Autodesk Inventor part; units mm, degrees
ref_plane "YZ Plane" through (0, 0, 0) normal (1, 0, 0) x (0, 1, 0)
ref_plane "XZ Plane" through (0, 0, 0) normal (0, 1, 0) x (-1, 0, 0)
ref_plane "XY Plane" through (0, 0, 0) normal (0, 0, 1) x (1, 0, 0)
sketch "Sketch2" plane through (0, 0, 0) normal (0, 0, 1) x (1, 0, 0)
  line L0 (-12.7, -30.6388) -> (12.7, -30.6388)
  line L1 (12.7, -30.6388) -> (12.7, 30.6388)
  line L2 (12.7, 30.6388) -> (-12.7, 30.6388)
  line L3 (-12.7, 30.6388) -> (-12.7, -30.6388)
  line L4 (-12.7, -30.6388) -> (12.7, 30.6388) construction
  line L5 (12.7, -30.6388) -> (-12.7, 30.6388) construction
  line L6 (0, 30.6388) -> (0, -30.6388) construction
  point P0 (0, 0)
  dimension "d0" = 25.4
  dimension "d1" = 61.2775
extrude "Extrusion1" add sketch "Sketch2" along normal blind 25.4
sketch "Sketch3" plane through (0, 0, 25.4) normal (0, 0, 1) x (1, 0, 0)
  line L0 (-12.7, -30.6388) -> (12.7, -30.6388) construction
  point P0 (0, 0)
  point P1 (0, -25.8762)
  dimension "d5" = 4.7625
hole "Hole1" at (0, -25.8762, 25.4) direction (0, 0, -1) diameter 4.826 end through all
fillet "Fillet1" radius 9.525 2 edges at (-12.7, -30.6388, 12.7) (12.7, -30.6388, 12.7)
pattern_linear "Rectangular Pattern1" count 5 spacing 12.7 along (0, 1, 0) of "Hole1"
sketch "Sketch4" plane through (0, 0, 25.4) normal (0, 0, 1) x (1, 0, 0)
  circle A0 centre (0, 24.9237) radius 2.413
  circle A1 centre (0, 12.2237) radius 2.413
  circle A2 centre (0, -0.4763) radius 2.413
  circle A3 centre (0, -13.1762) radius 2.413
  arc A4 (3.175, -30.6388) -> (12.7, -21.1137) centre (3.175, -21.1137) ccw
  line L0 (12.7, -21.1137) -> (12.7, 30.6388)
  line L1 (12.7, 30.6388) -> (-12.7, 30.6388)
  line L2 (-12.7, 30.6388) -> (-12.7, -21.1138)
  arc A5 (-12.7, -21.1138) -> (-3.175, -30.6388) centre (-3.175, -21.1138) ccw
  line L3 (-3.175, -30.6388) -> (3.175, -30.6388)
  circle A6 centre (0, -25.8762) radius 2.413
  circle A7 centre (0, -25.8762) radius 3.9688
  circle A8 centre (0, -13.1762) radius 3.9688
  circle A9 centre (0, -0.4763) radius 3.9688
  circle A10 centre (0, 12.2237) radius 3.9688
  circle A11 centre (0, 24.9237) radius 3.9688
  line L4 (2.413, -22.7253) -> (2.413, -16.3272)
  line L5 (2.413, -10.0253) -> (2.413, -3.6272)
  line L6 (-2.413, -22.7253) -> (-2.413, -16.3272)
  line L7 (-2.413, -10.0253) -> (-2.413, -3.6272)
  line L8 (2.413, 2.6747) -> (2.413, 9.0728)
  line L9 (-2.413, 2.6747) -> (-2.413, 9.0728)
  line L10 (-2.413, 15.3747) -> (-2.413, 21.7728)
  line L11 (2.413, 15.3747) -> (2.413, 21.7728)
  arc A12 (-10.668, -21.1138) -> (-3.175, -28.6068) centre (-3.175, -21.1138) ccw
  line L12 (-10.668, -21.1138) -> (-10.668, 28.6068)
  line L13 (-10.668, 28.6068) -> (10.668, 28.6068)
  line L14 (10.668, 28.6068) -> (10.668, -21.1137)
  arc A13 (3.175, -28.6068) -> (10.668, -21.1137) centre (3.175, -21.1137) ccw
  line L15 (3.175, -28.6068) -> (-3.175, -28.6068)
  point P0 (0, 0)
  point P1 (1.4787, 28.6068)
  point P2 (2.8802, -28.6068)
  point P3 (-2.8802, -28.6068)
  point P4 (-1.4787, 28.6068)
  dimension "d16" = 7.9375
  dimension "d17" = 2.032
extrude "Extrusion2" cut sketch "Sketch4" against normal through all contours A7 L4 A8 L5 A9 L8 A10 L11 A11 L13 L14 A13 L15 | A7 L15 A12 L12 L13 A11 L10 A10 L9 A9 L7 A8 L6
fillet "Fillet2" radius 3.175 21 edges at (2.8802, -28.6068, 12.7) (-2.8802, -28.6068, 12.7) (-1.4787, 28.6068, 12.7) (1.4787, 28.6068, 12.7) (-10.668, 28.6068, 12.7) (10.668, 28.6068, 12.7) (2.413, -16.3272, 12.7) (2.413, -10.0253, 12.7) (2.413, -3.6272, 12.7) (2.413, 2.6747, 12.7) (2.413, 9.0728, 12.7) (2.413, 15.3747, 12.7) (2.413, 21.7728, 12.7) (-2.413, -16.3272, 12.7) (-2.413, -10.0253, 12.7) (-2.413, -3.6272, 12.7) (-2.413, 2.6747, 12.7) (-2.413, 9.0728, 12.7) (-2.413, 15.3747, 12.7) (-2.413, 21.7728, 12.7) (-2.413, -22.7253, 12.7)
fillet "Fillet3" radius 4.7625 2 edges at (12.7, 30.6388, 12.7) (-12.7, 30.6388, 12.7)
properties part number "SDS LOWERING SPACER" material "Aluminum 7075"
The model under review builds one solid part; all positions refer to its coordinate system, in mm. A direction names the side the tool comes from. Round coordinates to 2 decimals unless told otherwise and drop trailing zeros. Order: outer loops, then holes, each group sorted by start corner. A loop starts at its lowest first (then second) coordinate and runs counter-clockwise, first axis right, second up. Notation, with made-up numbers: (63, 58) -> (117, 58) arc R20 ccw to (117, 93) -> close; hole circle Ø11 at (-21.5, 5). An arc over 180 degrees is marked (long way). Write item = value, one per line. Start each with the question number.
Item 1: For faces 4 (the face through (-3, 0, 0)), 5 (the face through (-2.6, 2.9, 12.5)), list the 3-axis set-ups (+Z, -Z, +X, -X, +Y, -Y) from which the entire face can be reached by the end or side of a thin tool; tool diameter is ignored.
Item 2: Consider section A-A on x = 0. Write out the cut boundary in (y, z), plus the area to 3 significant figures.
Item 3: Consider section C-C on z = 9.5. Count the separate pieces of the cut face and the enclosed holes in it, plus the area to 3 significant figures.
Item 4: Mouldability with a two-part tool opening along X and no side actions: class faces 1 (the face through (-11.27, 29.28, 12.88)), 2 (the face through (9.713, 27.701, 12.522)), 3 (the face through (9.84, -27.92, 12.88)) as released by +X, released by -X, zero draft, split by the parting line, or undercut.
Item 5: Consider section B-B on y = 14. Write out the cut boundary in (x, z), plus the area to 3 significant figures.
Item 6: For line 1 along X through (y, z) = (25, 14); line 2 along X through (y, z) = (6, 9.5); line 3 along Y through (x, z) = (0, 12.25), list the stretches that pass through material, from the lowest coordinate up.
Item 7: Clearance check with flat-ended pins moving along their axes: pin 1 Ø2 at (x, z) = (-10, 3.5) entering from -Y; pin 2 Ø1 at (x, z) = (10, 6) entering from +Y. State where each tip first meets the part, or that it passes through.
Conclusion:
q1.face_4 = -Z, +X, -X, +Y, -Y
q1.face_5 = +Z, -Z
q2.outline = (-30.64, 0) -> (-28.29, 0) -> (-28.29, 25.4) -> (-30.64, 25.4) -> close; (-23.46, 0) -> (-15.59, 0) -> (-15.59, 25.4) -> (-23.46, 25.4) -> close; (-10.76, 0) -> (-2.89, 0) -> (-2.89, 25.4) -> (-10.76, 25.4) -> close; (1.94, 0) -> (9.81, 0) -> (9.81, 25.4) -> (1.94, 25.4) -> close; (14.64, 0) -> (22.51, 0) -> (22.51, 25.4) -> (14.64, 25.4) -> close; (27.34, 0) -> (30.64, 0) -> (30.64, 25.4) -> (27.34, 25.4) -> close
q2.area = 944 mm2
q3.separate_pieces = 1
q3.enclosed_holes = 7
q3.area = 595 mm2
q4.face_1 = released by -X
q4.face_2 = undercut
q4.face_3 = released by +X
q5.outline = (-12.7, 0) -> (-10.67, 0) -> (-10.67, 25.4) -> (-12.7, 25.4) -> close; (-3.55, 0) -> (-1.63, 0) -> (-1.63, 25.4) -> (-3.55, 25.4) -> close; (1.63, 0) -> (3.55, 0) -> (3.55, 25.4) -> (1.63, 25.4) -> close; (10.67, 0) -> (12.7, 0) -> (12.7, 25.4) -> (10.67, 25.4) -> close
q5.area = 201 mm2
q6.line_1 = -12.7 to -10.67, -3.97 to -2.41, 2.41 to 3.97, 10.67 to 12.7
q6.line_2 = -12.7 to -10.67, -2.41 to 2.41, 10.67 to 12.7
q6.line_3 = -30.64 to -28.29, -23.46 to -15.59, -10.76 to -2.89, 1.94 to 9.81, 14.64 to 22.51, 27.34 to 30.64
q7.pin_1 = -28.65
q7.pin_2 = 30.38
